Could you check a few things on this model? Use its own coordinates, in mm. Give positions to 0.01 mm unless a question says otherwise; leave off trailing zeros. Loops run counter-clockwise (first coordinate to the right, second up) from the corner with the lowest first, then second, coordinate; pieces in that order, holes last. Notation, with made-up numbers: M 58,42 L 112,42 A8 cw 112,55 Z; hole C 49.25,86 d5. An arc over 180 degrees is marked long. Use a Markdown table: item, result. Add a question column.
1) Suppose I cut it at A-A on x = 19.5. List the corners of the cut face in (y, z) for me, and give its area (3 significant figures).
2) If I drill on line 1 along Z through (x, y) = (100, 1.5); line 2 along Z through (x, y) = (30.5, 4); line 3 along Z through (x, y) = (54, 2.5), over which ranges is the centre line in solid material (lowest first)? Write a range as [from, to].
3) Suppose I cut it at B-B on y = 1.25. List the corners of the cut face in (x, z) for me.
4) Will these pins go through, and if not, where does the flat tip stop? pin 1 Ø3 at (x, y) = (90, 2.5) entering from +Z; pin 2 Ø2 at (y, z) = (3, -68.5) entering from +X; pin 3 Ø2 at (y, z) = (3, -70) entering from -X.
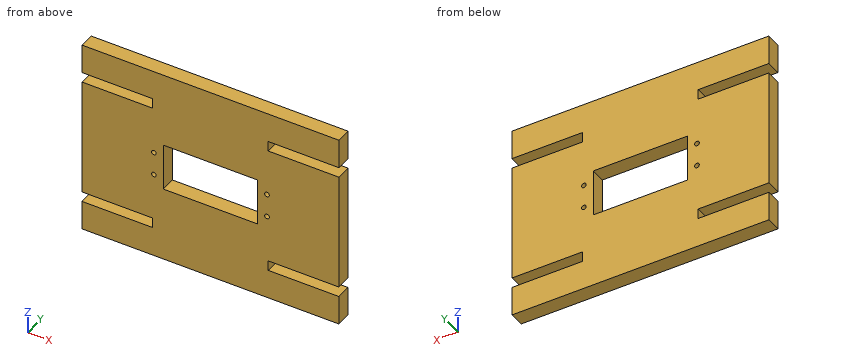
```python
from build123d import *

# Parameters (mm, degrees)
MAIN_SHAPE_DEPTH                            = 6.35
SKETCH2_W                                   = 40
SKETCH2_H                                   = 20
CUT_FOR_SERVO_MOUNTING_HOLE_LOCATIONS_DEPTH = 7.35
F_3_48_TAPPED_HOLE1_D                       = 1.9939
F_3_48_TAPPED_HOLE1_DEPTH                   = 7.67
F_3_48_TAPPED_HOLE1_TIP                     = 0.599027994


with BuildPart() as part:
    # Sketch1 → main shape (new body)
    with BuildSketch(Plane(origin=(0, 0, 0), x_dir=(1, 0, 0), z_dir=(0, 1, 0))):
        Polygon((0, 66.818), (0, 16.818), (30, 16.818), (30, 12.5), (0, 12.5), (0, 0), (109, 0), (109, 12.5), (79, 12.5), (79, 16.818), (109, 16.818), (109, 66.818), (79, 66.818), (79, 71.136), (109, 71.136), (109, 83.636), (0, 83.636), (0, 71.136), (30, 71.136), (30, 66.818), align=None)
    extrude(amount=MAIN_SHAPE_DEPTH)

    # Sketch2 → cut for servo + mounting hole locations (cut, through all)
    with BuildSketch(Plane(origin=(0, 6.35, 0), x_dir=(1, 0, 0), z_dir=(0, 1, 0))):
        with Locations((54.5, 41.818)):
            Rectangle(SKETCH2_W, SKETCH2_H)
    extrude(amount=-CUT_FOR_SERVO_MOUNTING_HOLE_LOCATIONS_DEPTH, mode=Mode.SUBTRACT)

    # #3-48 Tapped Hole1
    with Locations(Plane(origin=(0, 6.35, 0), x_dir=(-1, 0, 0), z_dir=(0, 1, 0))):
        with Locations((-30.5, -36.818), (-30.5, -46.818), (-78.5, -36.818), (-78.5, -46.818)):
            Hole(F_3_48_TAPPED_HOLE1_D / 2, depth=F_3_48_TAPPED_HOLE1_DEPTH)
            with Locations((0, 0, -(F_3_48_TAPPED_HOLE1_DEPTH + F_3_48_TAPPED_HOLE1_TIP / 2))):  # 118° drill point
                Cone(0, F_3_48_TAPPED_HOLE1_D / 2, F_3_48_TAPPED_HOLE1_TIP, mode=Mode.SUBTRACT)


solid = part.part
```
Answer block:
| question | item | result |
|---|---|---|
| 1 | outline | M 0,-83.64 L 6.35,-83.64 L 6.35,-71.14 L 0,-71.14 Z; M 0,-66.82 L 6.35,-66.82 L 6.35,-16.82 L 0,-16.82 Z; M 0,-12.5 L 6.35,-12.5 L 6.35,0 L 0,0 Z |
| 1 | area | 476 mm^2 |
| 2 | line 1 | z = [-83.64, -71.14], [-66.82, -16.82], [-12.5, 0] |
| 2 | line 2 | z = [-83.64, -47.81], [-45.82, -37.81], [-35.82, 0] |
| 2 | line 3 | z = [-83.64, -51.82], [-31.82, 0] |
| 3 | outline | M 0,-83.64 L 109,-83.64 L 109,-71.14 L 79,-71.14 L 79,-66.82 L 109,-66.82 L 109,-16.82 L 79,-16.82 L 79,-12.5 L 109,-12.5 L 109,0 L 0,0 L 0,-12.5 L 30,-12.5 L 30,-16.82 L 0,-16.82 L 0,-66.82 L 30,-66.82 L 30,-71.14 L 0,-71.14 Z; hole C 30.5,-46.82 d1.99; hole C 30.5,-36.82 d1.99; hole M 34.5,-51.82 L 74.5,-51.82 L 74.5,-31.82 L 34.5,-31.82 Z; hole C 78.5,-46.82 d1.99; hole C 78.5,-36.82 d1.99 |
| 4 | pin 1 | stops at z = 0 |
| 4 | pin 2 | stops at x = 79 |
| 4 | pin 3 | stops at x = 30 |
